Input: part model. Units: mm. Frame: model coordinates. A direction names the side the tool comes from. Give positions to 0.01 mm unless a question says otherwise; leave off trailing zeros. Loops run counter-clockwise (first coordinate to the right, second up) from the corner with the lowest first, then second, coordinate; pieces in that order, holes last. Notation, with made-up numbers: (-10, -11) - (29, -11) arc R7 ccw to (29, 1) - close; hole circle Ø11 at (34, -3). An arc over 180 degrees is marked (long way). One line per item, written item: value.
from build123d import *

# Parameters (mm, degrees)
F0_W      = 114.3
F0_H      = 114.3
F1_DEPTH  = 2.54
F8_W      = 114.3
F8_H      = 114.3
F9_DEPTH  = 2.54
F10_W     = 114.3
F10_H     = 114.3
F11_DEPTH = 2.54
F12_W     = 76.2
F12_H     = 104.14
F13_DEPTH = 1.27
F14_R     = 6.35
F15_DEPTH = 1.27
F17_W     = 111.252
F17_H     = 111.252
F18_DEPTH = 1.905


# Not quite as in the source:
# - a feature of the source that left no trace in its solid (it failed there, or was rolled back) is left out


with BuildPart() as f1:
    # F0 (on Top) → F1 (new body)
    with BuildSketch(Plane.XY):
        Rectangle(F0_W, F0_H)
    extrude(amount=F1_DEPTH)


with BuildPart() as f9:
    # F8 (on face) → F9 (new body)
    with BuildSketch(Plane.XY.offset(27.94)):
        Rectangle(F8_W, F8_H)
    extrude(amount=F9_DEPTH)

    # F10 (on face) → F11 (join)
    with BuildSketch(Plane.XY.offset(30.48)):
        Rectangle(F10_W, F10_H)
    extrude(amount=F11_DEPTH)

    # F12 (on face) → F13 (cut)
    with BuildSketch(Plane.XY.offset(33.02)):
        with Locations((-13.97, 0)):
            Rectangle(F12_W, F12_H)
    extrude(amount=-F13_DEPTH, mode=Mode.SUBTRACT)

    # F14 (on face) → F15 (cut)
    with BuildSketch(Plane.XY.offset(33.02)):
        with BuildLine():
            ThreePointArc((55.245, 45.72), (48.895, 52.07), (42.545, 45.72))
            ThreePointArc((42.545, 45.72), (48.895, 39.37), (55.245, 45.72))
        make_face()
        with Locations((32.385, 45.72)):
            Circle(F14_R)
        with BuildLine():
            ThreePointArc((40.64, 6.35), (36.1498719395, -4.4901280605), (46.99, 0))
            ThreePointArc((46.99, 0), (45.1301280605, 4.4901280605), (40.64, 6.35))
        make_face()
    extrude(amount=-F15_DEPTH, mode=Mode.SUBTRACT)


with BuildPart() as f18:
    # F17 (on face) → F18 (new body)
    with BuildSketch(Plane(origin=(0, 0, 27.94), x_dir=(1, 0, 0), z_dir=(0, 0, -1))):
        Rectangle(F17_W, F17_H)
    extrude(amount=F18_DEPTH)


solid = f9.part
Item 1: Access query for faces 1 (the face through (49, 46, 31.75)), 2 (the face through (25, -8, 33.02)). Directions: +Z, -Z, +X, -X, +Y, -Y. A direction counts if a zero-diameter tool reaches every point of the face in a straight line with its end or side. Return the directions, or none.
Verdict:
face 1: +Z
face 2: +Z, +X, -X, +Y, -Y
Item 2: Section B-B, the plane x = -34.5. Output: boundary loops of the cut face in (y, z).
Verdict:
outline: (-57.15, 27.94) - (57.15, 27.94) - (57.15, 33.02) - (52.07, 33.02) - (52.07, 31.75) - (-52.07, 31.75) - (-52.07, 33.02) - (-57.15, 33.02) - close
Item 3: Pin query (flat end, axial travel): P1, Ø10, axis at x = 48.895, y = 45.72, coming from the +Z side. Return the tip coordinate at first contact, or that it passes through.
Verdict:
P1: stops at z = 31.75
Item 4: Material intervals for L1, parallel to X at y = 0, z = 32.1; L2, parallel to Y at x = 2, z = 32.35; L3, parallel to Y at x = 40.64, z = 32.65, sorted ascending.
Verdict:
L1: x = -57.15 to -52.07, 24.13 to 34.29, 46.99 to 57.15
L2: y = -57.15 to -52.07, 52.07 to 57.15
L3: y = -57.15 to -6.35, 6.35 to 57.15
Item 5: Section A-A, the plane y = 26.5. Output: boundary loops of the cut face in (x, z), and give its area (3 significant figures).
Verdict:
outline: (-57.15, 27.94) - (57.15, 27.94) - (57.15, 33.02) - (24.13, 33.02) - (24.13, 31.75) - (-52.07, 31.75) - (-52.07, 33.02) - (-57.15, 33.02) - close
area: 484 mm^2
Item 6: Draft query along Y for faces 3 (the face through (32, 46, 31.75)), 4 (the face through (-1, -57.15, 30)), 5 (the face through (-1, 1, 27.94)). Return one class per face: pulls with the +Y half, pulls with the -Y half, needs draft (parallel to the pull), parting line crosses it, or undercut.
Verdict:
face 3: undercut
face 4: pulls with the -Y half
face 5: needs draft
Item 7: Section C-C, the plane y = 45.72. Output: boundary loops of the cut face in (x, z) (3 decimals).
Verdict:
outline: (-57.15, 27.94) - (57.15, 27.94) - (57.15, 33.02) - (55.245, 33.02) - (55.245, 31.75) - (42.545, 31.75) - (42.545, 33.02) - (38.735, 33.02) - (38.735, 31.75) - (26.035, 31.75) - (26.035, 33.02) - (24.13, 33.02) - (24.13, 31.75) - (-52.07, 31.75) - (-52.07, 33.02) - (-57.15, 33.02) - close
